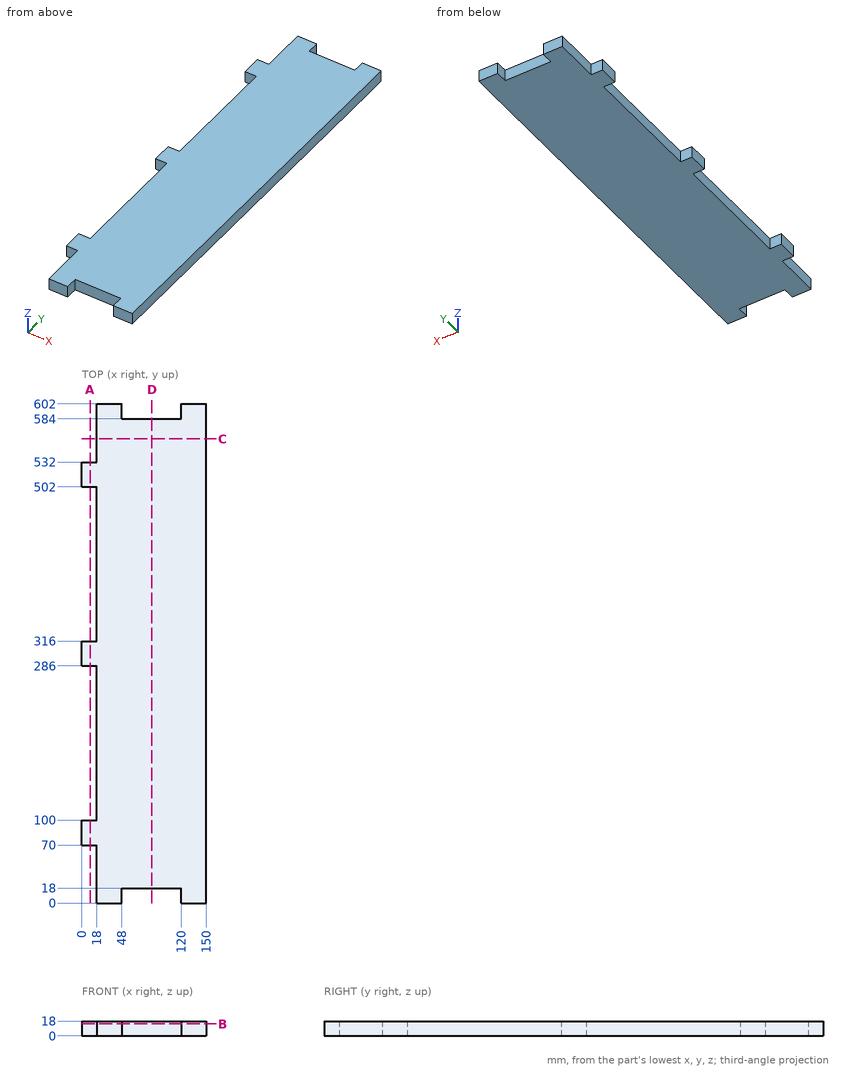
Here's the drawing with two shaded views (mm, measured from the low corner). I have some questions. Round coordinates to 2 decimals unless told otherwise and drop trailing zeros. Loops run counter-clockwise (first coordinate to the right, second up) from the corner with the lowest first, then second, coordinate; pieces in that order, holes last. Notation, with made-up numbers: M 37,-14.75 L 84,-14.75 A24 cw 84,0.25 Z; hole C 81.5,66 d11. An arc over 180 degrees is marked long. Answer as a JSON object with one key per item and string values. Group by question number.
Q1. Imagine slicing it at C-C, the plane y = 560. Please give me the cut outline in (x, z).
Q2. Imagine slicing it at D-D, the plane x = 84.5. Please give me the cut outline in (y, z), then the cut area to 3 significant figures.
Q3. Imagine slicing it at A-A, the plane x = 10. Please give me the cut outline in (y, z).
Q4. Imagine slicing it at B-B, the plane z = 14.75. Please give me the cut outline in (x, y).
Q5. Will these pins go through, and if not, where does the flat tip stop? pin 1 (5.5 mm diameter, centred on x = 12, z = 10.5, fed in from -Y); pin 2 (5.5 mm diameter, centred on y = 6.5, z = 4.5, fed in from -X); pin 3 (5 mm diameter, centred on x = 115, z = 12.5, fed in from +Y); pin 4 (5 mm diameter, centred on y = 85.5, z = 8, fed in from -X).
Q6. Please list where these lines run through material, in increasing order: L1, parallel to X at y = 189.5, z = 3.75; L2, parallel to Y at x = 67.5, z = 9.25.
Findings:
{
 "1": {"outline": "M 18,0 L 150,0 L 150,18 L 18,18 Z"},
 "2": {"outline": "M 18,0 L 584,0 L 584,18 L 18,18 Z", "area": "10,200 mm2"},
 "3": {"outline": "M 70,0 L 100,0 L 100,18 L 70,18 Z; M 286,0 L 316,0 L 316,18 L 286,18 Z; M 502,0 L 532,0 L 532,18 L 502,18 Z"},
 "4": {"outline": "M 0,70 L 18,70 L 18,0 L 48,0 L 48,18 L 120,18 L 120,0 L 150,0 L 150,602 L 120,602 L 120,584 L 48,584 L 48,602 L 18,602 L 18,532 L 0,532 L 0,502 L 18,502 L 18,316 L 0,316 L 0,286 L 18,286 L 18,100 L 0,100 Z"},
 "5": {"pin 1": "stops at y = 70", "pin 2": "stops at x = 18", "pin 3": "stops at y = 584", "pin 4": "stops at x = 0"},
 "6": {"L1": "x = 18 to 150", "L2": "y = 18 to 584"}
}
